The model under review builds one solid part; all positions refer to its coordinate system, in mm. A direction names the side the tool comes from. Coordinates: 2 decimals unless noted, no trailing zeros. Loops run counter-clockwise (first coordinate to the right, second up) from the corner with the lowest first, then second, coordinate; pieces in that order, holes last. Notation, with made-up numbers: M 51,-25.75 L 109,-25.75 A19 ccw 109,3.25 Z; hole C 39.25,41.25 d6. An arc over 180 degrees is marked long. Write item = value, one per line. Start each with the question number.
Q1. We need section B-B on z = -87.5. Give the boundary of the cut face in (x, y).
Q2. We need section C-C on x = -163.5. Give the boundary of the cut face in (y, z) (3 decimals), and give its area (3 significant figures).
Q3. We need section A-A on z = -97.5. Give the boundary of the cut face in (x, y).
Q4. Clearance check with flat-ended pins moving along their axes: pin 1 Ø12 at (y, z) = (15.5, -95.5) entering from +X; pin 2 Ø10 at (x, z) = (-137, -88) entering from +Y; pin 3 Ø17 at (x, z) = (-146.38, -89.11) entering from +Y. State where each tip first meets the part, or that it passes through.
Q5. Mouldability with a two-part tool opening along Z and no side actions: class faces 1 (the face through (-165, 50, -89)), 2 (the face through (-162, 18, -104.111)), 3 (the face through (-164.68, 15.97, -96.12)), 4 (the face through (-162, 18, -74.111)) as released by +Z, released by -Z, zero draft, split by the parting line, or undercut.
Q6. Wall thickness on probe 1 along Y at (x, z) = (-153, -81.75); probe 2 along X at (y, z) = (28.5, -97.25); probe 3 along Y at (x, z) = (-153, -86): over which ranges is each line inside the solid? List them lowest first.
Q7. For faces 5 (the face through (-137.452, 3.722, -90.283)), 6 (the face through (-168.084, 25, -89)), 7 (the face through (-159, 6.708, -96)), list the 3-axis set-ups (+Z, -Z, +X, -X, +Y, -Y) from which the entire face can be reached by the end or side of a thin tool; tool diameter is ignored.
Q8. We need section D-D on y = 24. Give the boundary of the cut face in (x, z), and give its area (3 significant figures).
from build123d import *

# Parameters (mm, degrees)
SKETCH2_W           = 30
SKETCH2_H           = 30
BOSS_EXTRUDE1_DEPTH = 6.708
SKETCH5_R           = 14
CUT_EXTRUDE1_DEPTH  = 2
SKETCH13_R          = 9
CUT_EXTRUDE3_DEPTH  = 2
SKETCH15_R          = 3
CUT_EXTRUDE5_DEPTH  = 8.35
SKETCH16_W          = 6.708000046
SKETCH16_H          = 50
BOSS_EXTRUDE3_DEPTH = 30
SKETCH17_R          = 1.7
CUT_EXTRUDE7_DEPTH  = 6.708


with BuildPart() as part:
    # Sketch2 → Boss-Extrude1 (new body)
    with BuildSketch(Plane(origin=(0, 0, 0), x_dir=(1, 0, 0), z_dir=(0, 1, 0))):
        with Locations((-146.375821197, 89.110918047)):
            Rectangle(SKETCH2_W, SKETCH2_H)
    extrude(amount=BOSS_EXTRUDE1_DEPTH)

    # Sketch5 → Cut-Extrude1 (cut)
    with BuildSketch(Plane(origin=(0, 6.708, 0), x_dir=(1, 0, 0), z_dir=(0, 1, 0))):
        with Locations(Location((-146.375821197, 89.110918047, 0), (0, 0, 270))):
            Circle(SKETCH5_R)
    extrude(amount=-CUT_EXTRUDE1_DEPTH, mode=Mode.SUBTRACT)

    # Sketch13 → Cut-Extrude3 (cut)
    with BuildSketch(Plane(origin=(0, 4.708, 0), x_dir=(1, 0, 0), z_dir=(0, 1, 0))):
        with Locations(Location((-146.375821197, 89.110918047, 0), (0, 0, 270))):
            Circle(SKETCH13_R)
    extrude(amount=-CUT_EXTRUDE3_DEPTH, mode=Mode.SUBTRACT)

    # Sketch15 → Cut-Extrude5 (cut)
    with BuildSketch(Plane(origin=(0, 2.708, 0), x_dir=(1, 0, 0), z_dir=(0, 1, 0))):
        with Locations(Location((-146.375821197, 89.110918047, 0), (0, 0, 270))):
            Circle(SKETCH15_R)
    extrude(amount=-CUT_EXTRUDE5_DEPTH, mode=Mode.SUBTRACT)

    # Sketch16 → Boss-Extrude3 (add)
    with BuildSketch(Plane.XY.offset(-74.110918047)):
        with Locations((-164.72982122, 25)):
            Rectangle(SKETCH16_W, SKETCH16_H)
    extrude(amount=-BOSS_EXTRUDE3_DEPTH)

    # Sketch17 → Cut-Extrude7 (cut)
    with BuildSketch(Plane(origin=(-161.375821197, 0, 0), x_dir=(0, 0, -1), z_dir=(1, 0, 0))):
        with Locations((81.610918047, 17.533)):
            Circle(SKETCH17_R)
        with Locations((96.490918047, 17.63)):
            Circle(SKETCH17_R)
        with Locations(Location((96.490918047, 39.078, 0), (0, 0, 180))):
            Circle(SKETCH17_R)
        with Locations(Location((81.610918047, 39.175, 0), (0, 0, 180))):
            Circle(SKETCH17_R)
    extrude(amount=-CUT_EXTRUDE7_DEPTH, mode=Mode.SUBTRACT)


solid = part.part
Returned:
q1.outline = M -168.08,0 L -148.91,0 L -148.91,2.71 L -155.23,2.71 L -155.23,4.71 L -160.28,4.71 L -160.28,6.71 L -161.38,6.71 L -161.38,50 L -168.08,50 Z; M -143.85,0 L -131.38,0 L -131.38,6.71 L -132.47,6.71 L -132.47,4.71 L -137.52,4.71 L -137.52,2.71 L -143.85,2.71 Z
q2.outline = M 0,-104.111 L 50,-104.111 L 50,-74.111 L 0,-74.111 Z; hole C 17.533,-81.611 d3.4; hole C 17.63,-96.491 d3.4; hole C 39.078,-96.491 d3.4; hole C 39.175,-81.611 d3.4
q2.area = 1,460 mm^2
q3.outline = M -168.08,0 L -131.38,0 L -131.38,6.71 L -135.17,6.71 L -135.17,4.71 L -143.12,4.71 L -143.12,2.71 L -149.64,2.71 L -149.64,4.71 L -157.58,4.71 L -157.58,6.71 L -161.38,6.71 L -161.38,16.26 L -168.08,16.26 Z; M -168.08,19 L -161.38,19 L -161.38,37.71 L -168.08,37.71 Z; M -168.08,40.45 L -161.38,40.45 L -161.38,50 L -168.08,50 Z
q4.pin_1 = -161.38
q4.pin_2 = 6.71
q4.pin_3 = 2.71
q5.face_1 = zero draft
q5.face_2 = released by -Z
q5.face_3 = undercut
q5.face_4 = released by +Z
q6.probe_1 = 0 to 4.71
q6.probe_2 = -168.08 to -161.38
q6.probe_3 = 0 to 2.71
q7.face_5 = +Y
q7.face_6 = +Z, -Z, -X, +Y, -Y
q7.face_7 = +Z, -Z, +X, +Y
q8.outline = M -168.08,-104.11 L -161.38,-104.11 L -161.38,-74.11 L -168.08,-74.11 Z
q8.area = 201 mm^2
